Read the model definition and answer for the solid it produces. Units are mm, in the model's axes. A direction names the side the tool comes from. Round coordinates to 2 decimals unless told otherwise and drop trailing zeros. Loops run counter-clockwise (first coordinate to the right, second up) from the corner with the lowest first, then second, coordinate; pieces in that order, holes last. Notation, with made-up numbers: (83, 56.5) -> (135, 56.5) arc R26 ccw to (135, 88.5) -> close; hole circle Ø6 at (66.5, -1). An arc over 180 degrees is marked (long way). Put each result on its own line as item: value.
from build123d import *

# Parameters (mm, degrees)
SKETCH4_W                  = 22.4536
SKETCH4_H                  = 22.4536
SKETCH4_W_2                = 20.066
SKETCH4_H_2                = 20.066
BOSS_EXTRUDE2_DEPTH        = 501.65
FILLET2_R                  = 3.81
FILLET1_R                  = 5.334
F_10_CLEARANCE_HOLE1_D     = 5.1054
F_10_CLEARANCE_HOLE1_DEPTH = 16.51
F_10_CLEARANCE_HOLE1_TIP   = 1.533816902
F_10_CLEARANCE_HOLE2_D     = 5.1054
CUT_EXTRUDE1_DEPTH         = 23.4536
CUT_EXTRUDE2_DEPTH         = 23.4536


with BuildPart() as part:
    # Sketch4 → Boss-Extrude2 (new body)
    with BuildSketch(Plane.XY):
        Rectangle(SKETCH4_W, SKETCH4_H)
        Rectangle(SKETCH4_W_2, SKETCH4_H_2, mode=Mode.SUBTRACT)
    extrude(amount=BOSS_EXTRUDE2_DEPTH)

    # Fillet2
    fillet2_edges = [part.edges().sort_by_distance(p)[0] for p in [
        (-10.033, 10.033, 250.825),
        (-10.033, -10.033, 250.825),
        (10.033, -10.033, 250.825),
        (10.033, 10.033, 250.825),
    ]]
    fillet(fillet2_edges, radius=FILLET2_R)

    # Fillet1
    fillet1_edges = [part.edges().sort_by_distance(p)[0] for p in [
        (-11.2268, 11.2268, 250.825),
        (11.2268, 11.2268, 250.825),
        (11.2268, -11.2268, 250.825),
        (-11.2268, -11.2268, 250.825),
    ]]
    fillet(fillet1_edges, radius=FILLET1_R)

    # #10 Clearance Hole1
    with Locations(Plane(origin=(0, 11.2268, 0), x_dir=(1, 0, 0), z_dir=(0, 1, 0))):
        with Locations((0, -12.7)):
            Hole(F_10_CLEARANCE_HOLE1_D / 2, depth=F_10_CLEARANCE_HOLE1_DEPTH)
            with Locations((0, 0, -(F_10_CLEARANCE_HOLE1_DEPTH + F_10_CLEARANCE_HOLE1_TIP / 2))):  # 118° drill point
                Cone(0, F_10_CLEARANCE_HOLE1_D / 2, F_10_CLEARANCE_HOLE1_TIP, mode=Mode.SUBTRACT)

    # #10 Clearance Hole2 (through all)
    with Locations(Plane(origin=(11.2268, 0, 0), x_dir=(0, 0, -1), z_dir=(1, 0, 0))):
        with Locations((-488.95, 0)):
            Hole(F_10_CLEARANCE_HOLE2_D / 2)

    # Sketch10 → Cut-Extrude1 (cut, through all)
    with BuildSketch(Plane.ZY.offset(11.2268)):
        Polygon((501.65, 11.2268), (491.179714367, -11.2268), (501.65, -11.2268), align=None)
    extrude(amount=-CUT_EXTRUDE1_DEPTH, mode=Mode.SUBTRACT)

    # Sketch11 → Cut-Extrude2 (cut, through all)
    with BuildSketch(Plane.ZY.offset(11.2268)):
        Polygon((501.65, 11.2268), (498.533209556, 11.2268), (501.093321918, 10.033), align=None)
    extrude(amount=-CUT_EXTRUDE2_DEPTH, mode=Mode.SUBTRACT)


solid = part.part
Item 1: A flat-ended cylindrical pin translates along its axis: pin 1 Ø4.5 at (y, z) = (0, 488.95) entering from +X. Find the tip coordinate at first contact, or state that the pin passes through.
Derived:
pin 1: passes through
Item 2: The part is cut by section A-A (z = 391). Determine the outline of the cut face in (x, y), then the cut area to 3 significant figures.
Derived:
outline: (-11.23, -5.89) arc R5.33 ccw to (-5.89, -11.23) -> (5.89, -11.23) arc R5.33 ccw to (11.23, -5.89) -> (11.23, 5.89) arc R5.33 ccw to (5.89, 11.23) -> (-5.89, 11.23) arc R5.33 ccw to (-11.23, 5.89) -> close; hole (-10.03, -6.22) arc R3.81 ccw to (-6.22, -10.03) -> (6.22, -10.03) arc R3.81 ccw to (10.03, -6.22) -> (10.03, 6.22) arc R3.81 ccw to (6.22, 10.03) -> (-6.22, 10.03) arc R3.81 ccw to (-10.03, 6.22) -> close
area: 89.6 mm^2
Item 3: For a pull along X with two mould halves and no side action, classify faces 3 (the flat face through (0, -10.033, 242)), 4 (the flat face through (11.227, 0, 246)), 5 (the flat face through (0, 11.227, 246)) as pulls with the +X half, pulls with the -X half, needs draft (parallel to the pull), parting line crosses it, or undercut.
Derived:
face 3: undercut
face 4: pulls with the +X half
face 5: needs draft
Item 4: Find the intervals of material crossed by line 1 along X through (y, z) = (-2.25, 37); line 2 along Z through (x, y) = (0, 10.9), in increasing order.
Derived:
line 1: x = -11.23 to -10.03, 10.03 to 11.23
line 2: z = 0 to 10.15, 15.25 to 499.23
Item 5: Which of the six approach directions +Z, -Z, +X, -X, +Y, -Y give full straight-line access (tool end or side, diameter ignored) to faces 1 (the flat face through (0, 10.033, 247)), 2 (the flat face through (0, -11, 0))?
Derived:
face 1: +Z, -Z
face 2: -Z, +X, -X, +Y, -Y
